from build123d import *

# Parameters (mm, degrees)
F0_R     = 15
F1_DEPTH = 30
F2_R     = 12.5
F3_DEPTH = 25
F4_W     = 12.5
F4_H     = 12.5
F5_DEPTH = 5.001


with BuildPart() as f1:
    # F0 (on Top) → F1 (new body)
    with BuildSketch(Plane.XY):
        Circle(F0_R)
    extrude(amount=F1_DEPTH)

    # F2 (on face) → F3 (cut)
    with BuildSketch(Plane.XY.offset(30)):
        Circle(F2_R)
    extrude(amount=-F3_DEPTH, mode=Mode.SUBTRACT)

    # F4 (on face) → F5 (cut, through all)
    with BuildSketch(Plane.XY.offset(5)):
        Rectangle(F4_W, F4_H)
    extrude(amount=-F5_DEPTH, mode=Mode.SUBTRACT)


solid = f1.part
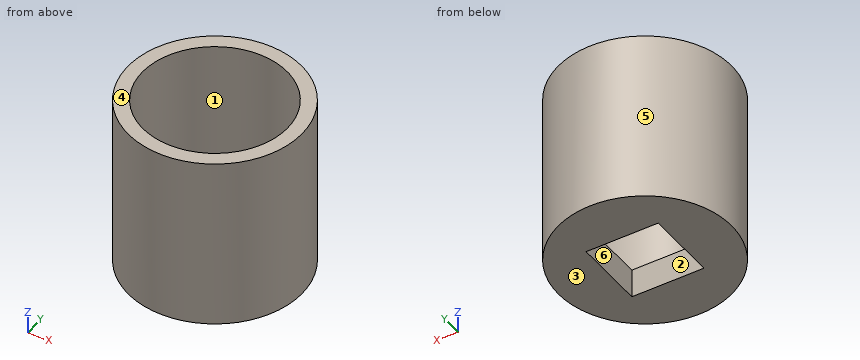
Here's how the part is built. I have some questions about the finished solid (model axes, mm). Face numbers are marked on the shaded views. A direction names the side the tool comes from. Give positions to 0.01 mm unless a question says otherwise; leave off trailing zeros. Write each loop counter-clockwise with the first axis right and the second up, starting at its lowest first coordinate (ties: lowest second). Pieces come first, ordered by that corner, then holes. Notation, with made-up numbers: (55.5, 2) -> (65.5, 2) arc R36 cw to (65.5, 41) -> close; hole circle Ø4 at (-39.5, 85). An arc over 180 degrees is marked (long way). Use one line per item in the form item = value. Start each with the question number.
1. Will these pins go through, and if not, where does the flat tip stop? pin 1 Ø3 at (x, y) = (0.5, -7.5) entering from +Z; pin 2 Ø10 at (y, z) = (-6, 7.5) entering from -X; pin 3 Ø2 at (x, z) = (9, 25) entering from -Y.
2. On a 3-axis mill with a long thin cutter (end or side, diameter ignored), from which of +Z, -Z, +X, -X, +Y, -Y can I reach the whole of each face in a straight line? I mean the marked faces 1, 2 and 3. Say none if no direction works.
3. Imagine slicing it at C-C on y = 9. List the corners of the cut face in (x, z) for me.
4. Thinking about a two-plate mould opening in Y: for the marked faces 4, 5 and 6, which applies, +Y half, -Y half, draft (parallel to the pull), parting line (faces both ways), or undercut?
5. Imagine slicing it at A-A on y = 0. List the corners of the cut face in (x, z) for me.
6. If I drill on L1, parallel to Y at x = 0, z = 18.5; L2, parallel to Y at x = 8, z = 27; L3, parallel to X at y = 10.5, z = 5.75, over which ranges is the centre line in solid material (lowest first)?
7. Imagine slicing it at D-D on z = 7.5. List the corners of the cut face in (x, y) for me, plus the area to 3 significant figures.
Entries:
q1.pin_1 = 5
q1.pin_2 = -14.97
q1.pin_3 = -12.69
q2.face_1 = +Z
q2.face_2 = +Z, -Z
q2.face_3 = -Z, +X, -X, +Y, -Y
q3.outline = (-12, 0) -> (12, 0) -> (12, 30) -> (8.67, 30) -> (8.67, 5) -> (-8.67, 5) -> (-8.67, 30) -> (-12, 30) -> close
q4.face_4 = draft
q4.face_5 = parting line
q4.face_6 = undercut
q5.outline = (-15, 0) -> (-6.25, 0) -> (-6.25, 5) -> (-12.5, 5) -> (-12.5, 30) -> (-15, 30) -> close; (6.25, 0) -> (15, 0) -> (15, 30) -> (12.5, 30) -> (12.5, 5) -> (6.25, 5) -> close
q6.L1 = -15 to -12.5, 12.5 to 15
q6.L2 = -12.69 to -9.6, 9.6 to 12.69
q6.L3 = -10.71 to -6.78, 6.78 to 10.71
q7.outline = circle Ø30 at (0, 0); hole circle Ø25 at (0, 0)
q7.area = 216 mm²
